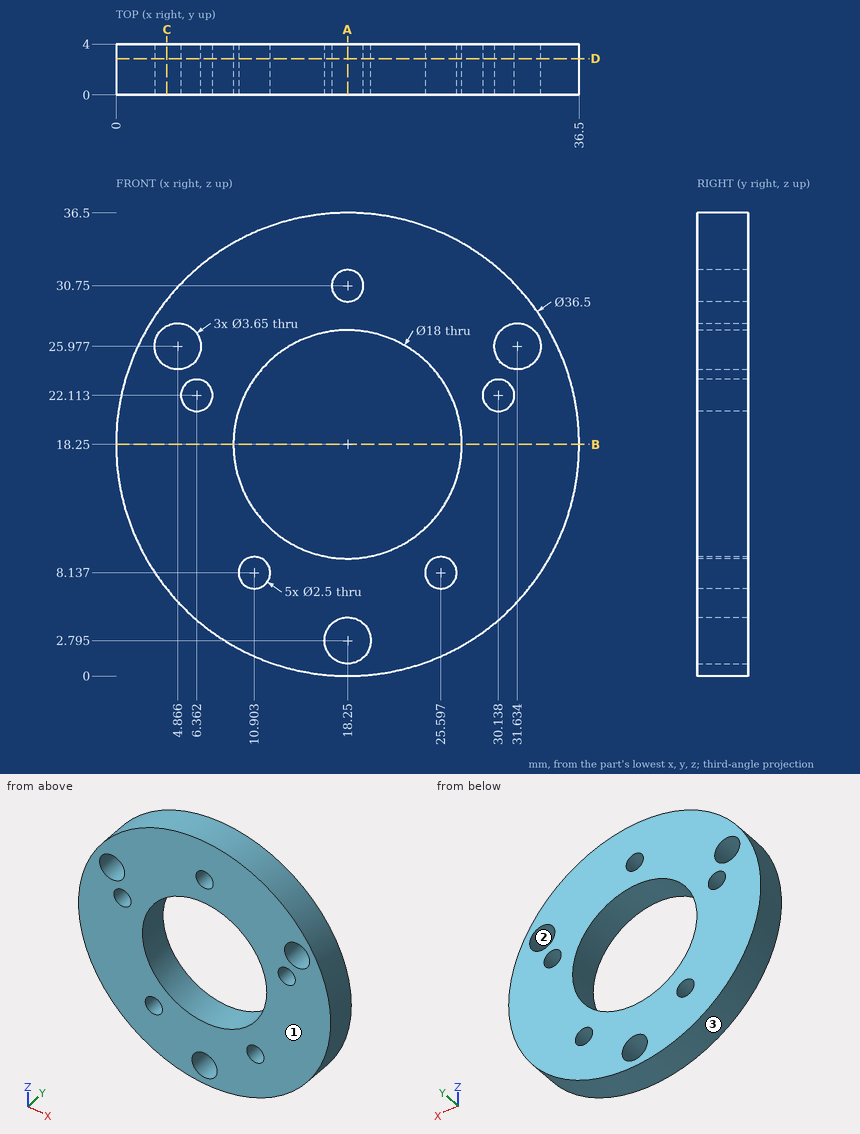
Here's the drawing with two shaded views (mm, measured from the low corner). I have some questions. Round coordinates to 2 decimals unless told otherwise and drop trailing zeros. Order: outer loops, then holes, each group sorted by start corner. A loop starts at its lowest first (then second) coordinate and runs counter-clockwise, first axis right, second up. Notation, with made-up numbers: M 62.5,-24.5 L 114.5,-24.5 A30 ccw 114.5,-0.5 Z; hole C 7.25,66 d4. An arc over 180 degrees is marked long. Answer in a Markdown table with one row per item.
Item 1: Thinking about a two-plate mould opening in X: for the marked faces 1, 2 and 3, which applies, +X half, -X half, draft (parallel to the pull), parting line (faces both ways), or undercut?
A:
| item | result |
|---|---|
| face 1 | draft |
| face 2 | undercut |
| face 3 | parting line |
Item 2: Imagine slicing it at D-D, the plane y = 2.85. State how many separate pieces and enclosed holes the cut face has, and give its area (3 significant figures).
A:
| item | result |
|---|---|
| separate pieces | 1 |
| enclosed holes | 9 |
| area | 736 mm2 |
Item 3: Imagine slicing it at A-A, the plane x = 18.25. Write out the boundary of the cut face in (y, z).
A:
| item | result |
|---|---|
| outline | M 0,0 L 4,0 L 4,0.97 L 0,0.97 Z; M 0,4.62 L 4,4.62 L 4,9.25 L 0,9.25 Z; M 0,27.25 L 4,27.25 L 4,29.5 L 0,29.5 Z; M 0,32 L 4,32 L 4,36.5 L 0,36.5 Z |
Item 4: Imagine slicing it at B-B, the plane z = 18.25. Write out the boundary of the cut face in (x, y).
A:
| item | result |
|---|---|
| outline | M 0,0 L 9.25,0 L 9.25,4 L 0,4 Z; M 27.25,0 L 36.5,0 L 36.5,4 L 27.25,4 Z |
Item 5: I'm going to push a flat-ended pin straight in: pin 1 (1 mm diameter, centred on y = 3, z = 9.5, fed in from -X). Where does the tip first touch, or does it pass through?
A:
| item | result |
|---|---|
| pin 1 | stops at x = 1.97 |
Item 6: Imagine slicing it at C-C, the plane x = 4. Write out the boundary of the cut face in (y, z).
A:
| item | result |
|---|---|
| outline | M 0,6.85 L 4,6.85 L 4,24.37 L 0,24.37 Z; M 0,27.58 L 4,27.58 L 4,29.65 L 0,29.65 Z |
Item 7: If I drill on L1, parallel to Z at x = 18.25, y = 2.85; L2, parallel to X at y = 1.6, z = 22; L3, parallel to Z at x = 25.5, y = 0.9 (1 decimal), over which ranges is the centre line in solid material (lowest first)? Write a range as from..to.
A:
| item | result |
|---|---|
| L1 | z = 0..0.97, 4.62..9.25, 27.25..29.5, 32..36.5 |
| L2 | x = 0.39..5.12, 7.61..10.07, 26.43..28.89, 31.38..36.11 |
| L3 | z = 1.5..6.9, 9.4..12.9, 23.6..35 |
